Check sheet for the drawn part. Datum: minimum x, y, z corner. Units: mm. Round coordinates to 2 decimals unless told otherwise and drop trailing zeros. One line per item, written item: value.
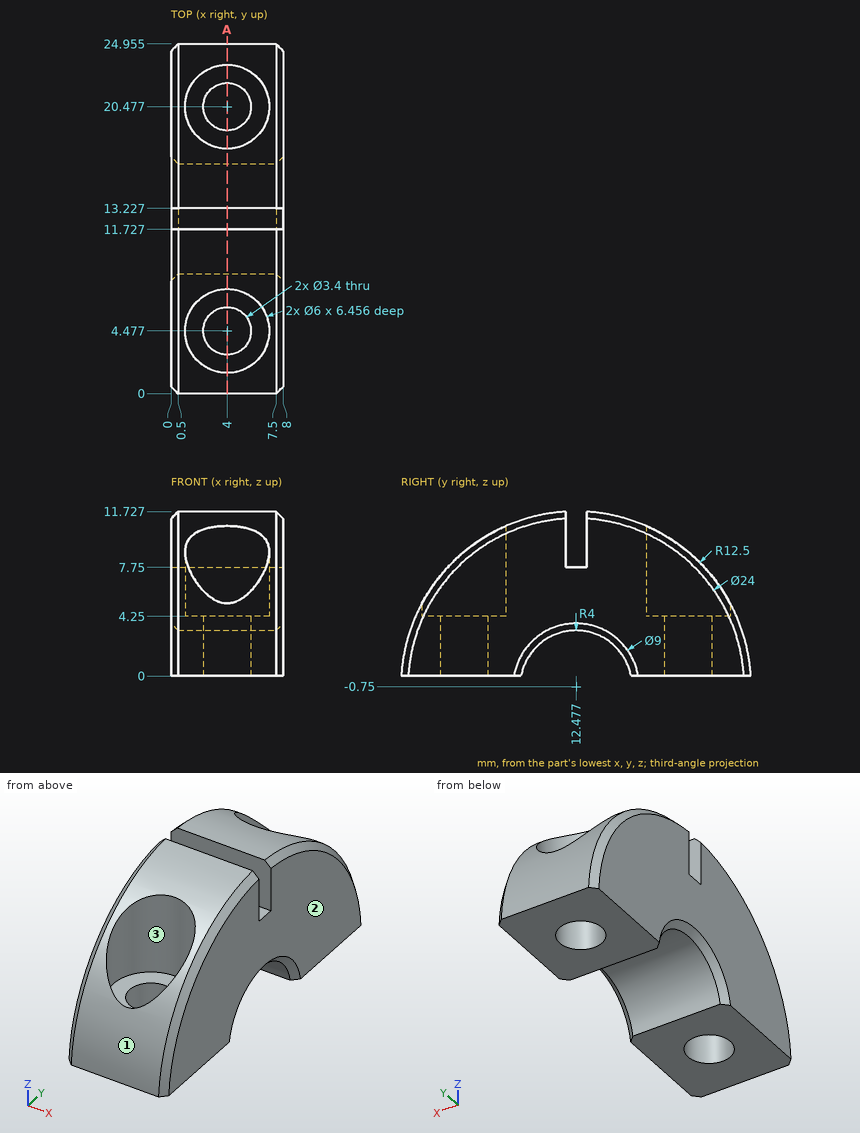
Q1. Sectioned sample at A-A on x = 4. State how many separate pieces and enclosed holes the cut face has, and give its area (3 significant figures).
Completed:
separate pieces: 3
enclosed holes: 0
area: 121 mm^2
Q2. Draft check along Y on the marked faces 1, 2 and 3. Enter one of: pulls with the +Y half, pulls with the -Y half, needs draft (parallel to the pull), parting line crosses it, or undercut.
Completed:
face 1: pulls with the -Y half
face 2: needs draft
face 3: undercut
Q3. Depth check by flat-ended pin: P1, Ø4.5, axis at x = 4.5, z = 9.5, coming from the +Y side (1 decimal); P2, Ø4.5, axis at x = 4, y = 20.48, coming from the +Z side; P3, Ø3, axis at x = 2, z = 10, coming from the -Y side. Enter the tip coordinate at first touch or a pass-through.
Completed:
P1: y = 19.3
P2: z = 4.25
P3: y = 4.51
Q4. Scan lines: line 1 (Z direction, x = 5, y = 2); line 2 (Y direction, x = 3.75, z = 1) (1 decimal); line 3 (X direction, y = 7, z = 5.25) (1 decimal). Record each from-to range of solid material in increasing order. Write a range as [from, to].
Completed:
line 1: [0, 4.25]
line 2: [0.1, 2.8], [6.2, 8.9], [16.1, 18.8], [22.2, 24.9]
line 3: [0, 2.4], [5.6, 8]
